Verification items for the finished model (mm, model axes). A direction names the side the tool comes from. Round coordinates to 2 decimals unless told otherwise and drop trailing zeros. Write each loop counter-clockwise with the first axis right and the second up, starting at its lowest first coordinate (ties: lowest second). Pieces come first, ordered by that corner, then holes. Notation, with made-up numbers: M 29.25,25 L 86.25,25 A11 cw 86.25,39 Z; hole C -4.5,14 d8. An arc over 180 degrees is marked long. Answer in a Markdown table with one row per item. Add a question column.
1. Sectioned sample at A-A on z = -30.5. Record the cut outline in (x, y), plus the area to 3 significant figures.
2. Sectioned sample at B-B on z = -4. Record the cut outline in (x, y), plus the area to 3 significant figures.
3. Sectioned sample at C-C on x = 0. Record the cut outline in (y, z), plus the area to 3 significant figures.
4. Go/stop test with flat-tipped pins: pin 1 Ø2.5 at (x, y) = (-67.5, 5) entering from -Z; pin 2 Ø6 at (x, z) = (5, -14.5) entering from +Y; pin 3 Ø6 at (y, z) = (-2, -26.5) entering from +X; pin 4 Ø6.5 at (x, z) = (-39.5, -3) entering from -Y. Record where each tip stops, or that it passes through.
5. Sectioned sample at D-D on x = 40. Record the cut outline in (y, z), plus the area to 3 significant figures.
6. Draft check along X on faces 1 (the flat face through (-114, -26, -38)), 2 (the flat face through (-175, -37, -16)), 3 (the flat face through (-76, -50, -9)). Enter one of: pulls with the +X half, pulls with the -X half, needs draft (parallel to the pull), parting line crosses it, or undercut.
7. Set-up check for faces 4 (the flat face through (-113, 25, -7)), 5 (the flat face through (-48, -90, -1)), 6 (the cylindrical face through (-84.01, -62.15, -6.66)), 7 (the cylindrical face through (14.063, 69.593, -9.126)): record each of +Z, -Z, +X, -X, +Y, -Y from which the full face is reachable in a straight line by a thin tool's end or side.
8. Material ranges on probe 1 along Y at (x, z) = (-91, -33.75); probe 2 along Y at (x, z) = (-67, 2); probe 3 along Z at (x, y) = (35.5, -32), recorded low to high.
```python
from build123d import *

# Parameters (mm, degrees)
BOSS_EXTRUDE8_DEPTH  = 5
SKETCH18_W           = 250
SKETCH18_H           = 15
BOSS_EXTRUDE9_DEPTH  = 8
SKETCH19_R           = 22.5
SKETCH19_R_2         = 2
CUT_EXTRUDE4_DEPTH   = 8
SKETCH20_R           = 2
CUT_EXTRUDE5_DEPTH   = 8
BOSS_EXTRUDE11_START = 18
BOSS_EXTRUDE11_DEPTH = 18
SKETCH22_W           = 104
SKETCH22_H           = 15.211863575
BOSS_EXTRUDE12_DEPTH = 10
CUT_EXTRUDE6_DEPTH   = 10
BOSS_EXTRUDE13_DEPTH = 20
SKETCH26_R           = 4
CUT_EXTRUDE7_DEPTH   = 30
SKETCH27_W           = 4
SKETCH27_H           = 15
CUT_EXTRUDE8_DEPTH   = 10


# Read off the part's stored shape, not the designer's step: Boss-Extrude13
with BuildPart() as part:
    # Sketch13 → Boss-Extrude8 (new body)
    with BuildSketch(Plane.XY):
        with BuildLine():
            Line((-167.919375153, 27.161249695), (-21.895313644, 71.732804493))
            ThreePointArc((-21.895313644, 71.732804493), (44.625393425, 60.279136205), (75, 0))
            Line((75, 0), (75, -75))
            Line((75, -75), (75, -90))
            Line((75, -90), (-175, -90))
            Line((-175, -90), (-175, -75))
            Line((-175, -75), (-175, 17.596875763))
            ThreePointArc((-175, 17.596875763), (-173.037218161, 23.546928219), (-167.919375153, 27.161249695))
        make_face()
    extrude(amount=BOSS_EXTRUDE8_DEPTH)

    # Sketch18 → Boss-Extrude9 (add)
    with BuildSketch(Plane(origin=(0, 0, 0), x_dir=(-1, 0, 0), z_dir=(0, 0, -1))):
        with Locations((50, -82.5)):
            Rectangle(SKETCH18_W, SKETCH18_H)
    extrude(amount=BOSS_EXTRUDE9_DEPTH)

    # Sketch19 → Cut-Extrude4 (cut)
    with BuildSketch(Plane(origin=(0, 0, 0), x_dir=(-1, 0, 0), z_dir=(0, 0, -1))):
        Circle(SKETCH19_R)
        with Locations((-67.5, -65)):
            Circle(SKETCH19_R_2)
        with Locations((67.5, -65)):
            Circle(SKETCH19_R_2)
        with Locations((67.5, -30)):
            Circle(SKETCH19_R_2)
        with Locations((67.5, 5)):
            Circle(SKETCH19_R_2)
        with Locations((-67.5, -30)):
            Circle(SKETCH19_R_2)
        with Locations((-67.5, 5)):
            Circle(SKETCH19_R_2)
    extrude(amount=-CUT_EXTRUDE4_DEPTH, mode=Mode.SUBTRACT)

    # Sketch20 → Cut-Extrude5 (cut)
    with BuildSketch(Plane(origin=(0, 0, 0), x_dir=(-1, 0, 0), z_dir=(0, 0, -1))):
        with Locations((-45, 50)):
            Circle(SKETCH20_R)
        with Locations((45, 50)):
            Circle(SKETCH20_R)
    extrude(amount=-CUT_EXTRUDE5_DEPTH, mode=Mode.SUBTRACT)

    # Sketch21 → Boss-Extrude11 (add)
    with BuildSketch(Plane(origin=(0, 0, 0), x_dir=(-1, 0, 0), z_dir=(0, 0, -1)).offset(BOSS_EXTRUDE11_START)):
        with BuildLine():
            Line((167.919375153, 27.161249695), (21.895313644, 71.732804493))
            ThreePointArc((21.895313644, 71.732804493), (51.864787491, 54.176044692), (70.710678119, 25))
            Line((70.710678119, 25), (91, 25))
            Line((91, 25), (161, 25))
            ThreePointArc((161, 25), (168.071067812, 22.071067812), (171, 15))
            Line((171, 15), (171, -55))
            ThreePointArc((171, -55), (168.071067812, -62.071067812), (161, -65))
            Line((161, -65), (91, -65))
            ThreePointArc((91, -65), (83.928932188, -62.071067812), (81, -55))
            Line((81, -55), (81, -50))
            Line((81, -50), (71, -50))
            Line((71, -50), (71, -75))
            Line((71, -75), (75, -75))
            Line((75, -75), (85, -75))
            Line((85, -75), (175, -75))
            Line((175, -75), (175, 17.596875763))
            ThreePointArc((175, 17.596875763), (173.037218161, 23.546928219), (167.919375153, 27.161249695))
        make_face()
        with BuildLine():
            ThreePointArc((21.895313644, 71.732804493), (-44.625393425, 60.279136205), (-75, 0))
            Line((-75, 0), (-75, -75))
            Line((-75, -75), (-71, -75))
            Line((-71, -75), (-71, 0))
            ThreePointArc((-71, 0), (-12.705070757, 69.853999006), (66.452990903, 25))
            Line((66.452990903, 25), (70.710678119, 25))
            ThreePointArc((70.710678119, 25), (51.864787491, 54.176044692), (21.895313644, 71.732804493))
        make_face()
    extrude(amount=-BOSS_EXTRUDE11_DEPTH)

    # Sketch22 → Boss-Extrude12 (add)
    with BuildSketch(Plane(origin=(0, 0, -8), x_dir=(-1, 0, 0), z_dir=(0, 0, -1))):
        with Locations((123, -82.605931787)):
            Rectangle(SKETCH22_W, SKETCH22_H)
    extrude(amount=BOSS_EXTRUDE12_DEPTH)

    # Sketch24 → Cut-Extrude6 (cut)
    with BuildSketch(Plane(origin=(0, 0, 0), x_dir=(-1, 0, 0), z_dir=(0, 0, -1))):
        with BuildLine():
            Line((91, 25), (161, 25))
            ThreePointArc((161, 25), (168.071067812, 22.071067812), (171, 15))
            Line((171, 15), (171, -55))
            ThreePointArc((171, -55), (168.071067812, -62.071067812), (161, -65))
            Line((161, -65), (91, -65))
            ThreePointArc((91, -65), (83.928932188, -62.071067812), (81, -55))
            Line((81, -55), (81, 15))
            ThreePointArc((81, 15), (83.928932188, 22.071067812), (91, 25))
        make_face()
    extrude(amount=-CUT_EXTRUDE6_DEPTH, mode=Mode.SUBTRACT)

    # Boss-Extrude13 outline → Boss-Extrude13 (add)
    with BuildSketch(Plane(origin=(0, 0, -18), x_dir=(-1, 0, 0), z_dir=(0, 0, -1))):
        with BuildLine():
            Line((175, -90.211863575), (175, 17.394801859))
            ThreePointArc((175, 17.394801859), (173.040981021, 23.339768152), (167.931475155, 26.955474085))
            Line((167.931475155, 26.955474085), (22.076778478, 71.67716409))
            ThreePointArc((22.076778478, 71.67716409), (60.335554965, 44.549083123), (75, 0))
            Line((75, 0), (75, -90.211863575))
            Line((75, -90.211863575), (175, -90.211863575))
        make_face()
    extrude(amount=BOSS_EXTRUDE13_DEPTH)

    # Sketch26 → Cut-Extrude7 (cut)
    with BuildSketch(Plane(origin=(0, 0, -38), x_dir=(-1, 0, 0), z_dir=(0, 0, -1))):
        with Locations((161, 15)):
            Circle(SKETCH26_R)
        with Locations((91, 15)):
            Circle(SKETCH26_R)
        with Locations((91, -55)):
            Circle(SKETCH26_R)
        with Locations((161, -55)):
            Circle(SKETCH26_R)
    extrude(amount=-CUT_EXTRUDE7_DEPTH, mode=Mode.SUBTRACT)

    # Sketch27 → Cut-Extrude8 (cut)
    with BuildSketch(Plane(origin=(0, 0, -18), x_dir=(-1, 0, 0), z_dir=(0, 0, -1))):
        with Locations((73, -82.711863575)):
            Rectangle(SKETCH27_W, SKETCH27_H)
    extrude(amount=-CUT_EXTRUDE8_DEPTH, mode=Mode.SUBTRACT)


solid = part.part
```
Geometry check:
| question | item | result |
|---|---|---|
| 1 | outline | M -175,-90.21 L -75,-90.21 L -75,0 A75 cw -22.08,71.68 L -167.93,26.96 A10 ccw -175,17.39 Z; hole C -161,-55 d8; hole C -161,15 d8; hole C -91,-55 d8; hole C -91,15 d8 |
| 1 | area | 13,400 mm2 |
| 2 | outline | M -175,-90 L 75,-90 L 75,0 A75 ccw -21.9,71.73 L -167.92,27.16 A10 ccw -175,17.6 Z; hole M -171,-55 A10 ccw -161,-65 L -91,-65 A10 ccw -81,-55 L -81,-50 L -71,-50 L -71,-75 L 71,-75 L 71,0 A71 ccw -66.45,25 L -161,25 A10 ccw -171,15 Z |
| 2 | area | 8,540 mm2 |
| 3 | outline | M -90,-8 L -75,-8 L -75,0 L -22.5,0 L -22.5,5 L -90,5 Z; M 22.5,0 L 71,0 L 71,-18 L 75,-18 L 75,5 L 22.5,5 Z |
| 3 | area | 792 mm2 |
| 4 | pin 1 | passes through |
| 4 | pin 2 | stops at y = 74.97 |
| 4 | pin 3 | stops at x = -74.99 |
| 4 | pin 4 | stops at y = -90 |
| 5 | outline | M -90,-8 L -75,-8 L -75,0 L 58.66,0 L 58.66,-18 L 63.44,-18 L 63.44,5 L -90,5 Z |
| 5 | area | 973 mm2 |
| 6 | face 1 | needs draft |
| 6 | face 2 | pulls with the -X half |
| 6 | face 3 | undercut |
| 7 | face 4 | none |
| 7 | face 5 | +Z, +X, -X, -Y |
| 7 | face 6 | +Z |
| 7 | face 7 | -Z |
| 8 | probe 1 | y = -90.21 to -59, -51 to 11, 19 to 50.54 |
| 8 | probe 2 | y = -90 to -66.94, -63.06 to -31.94, -28.06 to 3.06, 6.94 to 57.97 |
| 8 | probe 3 | z = 0 to 5 |
